The listing builds one solid part. Answer for the finished solid, in the listing's coordinates (mm). Face numbers are marked on the shaded views. A direction names the side the tool comes from. Round coordinates to 2 decimals unless told otherwise and drop trailing zeros. Loops run counter-clockwise (first coordinate to the right, second up) from the corner with the lowest first, then second, coordinate; pieces in that order, holes last. Notation, with made-up numbers: (19, -20.75) -> (52, -20.75) arc R30 ccw to (52, 4.25) -> close; hole circle Ø7 at (-1, 78). An arc over 180 degrees is marked (long way). One line per question, with ' | ' between items.
from build123d import *

# Parameters (mm, degrees)
SKETCH5_R           = 30
BOSS_EXTRUDE1_DEPTH = 5
SKETCH6_R           = 5.75
CUT_EXTRUDE1_DEPTH  = 50
SKETCH11_R          = 1.5
CUT_EXTRUDE2_DEPTH  = 43.720018727
SKETCH13_R          = 1.5
CUT_EXTRUDE3_DEPTH  = 10
CIRPATTERN2_COUNT   = 6
CUT_EXTRUDE4_DEPTH  = 10


with BuildPart() as part:
    # Sketch5 → Boss-Extrude1 (new body)
    with BuildSketch(Plane(origin=(0, 0, 0), x_dir=(1, 0, 0), z_dir=(0, 1, 0))):
        with Locations(Location((0, 0, 0), (0, 0, 270))):
            Circle(SKETCH5_R)
    extrude(amount=BOSS_EXTRUDE1_DEPTH)

    # Sketch6 → Cut-Extrude1 (cut)
    with BuildSketch(Plane(origin=(0, 5, 0), x_dir=(1, 0, 0), z_dir=(0, 1, 0))):
        with Locations(Location((5.564652455, 9.430649132, 0), (0, 0, 270))):
            Circle(SKETCH6_R)
        with Locations(Location((5.325305202, -9.567843252, 0), (0, 0, 270))):
            Circle(SKETCH6_R)
        with Locations(Location((-11.00819821, 0.138683741, 0), (0, 0, 270))):
            Circle(SKETCH6_R)
    extrude(amount=-CUT_EXTRUDE1_DEPTH, mode=Mode.SUBTRACT)

    # Sketch11 → Cut-Extrude2 (cut, through all)
    with BuildSketch(Plane(origin=(0, 5, 0), x_dir=(1, 0, 0), z_dir=(0, 1, 0))):
        with Locations(Location((0, 0, 0), (0, 0, 270))):
            Circle(SKETCH11_R)
    extrude(amount=-CUT_EXTRUDE2_DEPTH, mode=Mode.SUBTRACT)

    # Sketch13 → Cut-Extrude3 (cut)
    with BuildSketch(Plane(origin=(0, 5, 0), x_dir=(1, 0, 0), z_dir=(0, 1, 0))):
        with Locations(Location((0, 25, 0), (0, 0, 270))):
            Circle(SKETCH13_R)
    cut_extrude3 = extrude(amount=-CUT_EXTRUDE3_DEPTH, mode=Mode.SUBTRACT)

    # CirPattern2: Cut-Extrude3 ×6 about axis
    cirpattern2_axis = Axis((0, 0, 0), (0, 1, 0))
    for i in range(1, CIRPATTERN2_COUNT):
        add(cut_extrude3.rotate(cirpattern2_axis, i * 360 / CIRPATTERN2_COUNT), mode=Mode.SUBTRACT)

    # Sketch14 → Cut-Extrude4 (cut)
    with BuildSketch(Plane(origin=(0, 5, 0), x_dir=(1, 0, 0), z_dir=(0, 1, 0))):
        with BuildLine():
            Line((9.868938528, -7.038931193), (19.133510592, -23.684357125))
            ThreePointArc((19.133510592, -23.684357125), (17.118789327, -30.75690251), (10.046243942, -28.742181244))
            Line((10.046243942, -28.742181244), (0.781671877, -12.096755312))
            ThreePointArc((0.781671877, -12.096755312), (2.796393143, -5.024209927), (9.868938528, -7.038931193))
        make_face()
        with BuildLine():
            Line((1.086170675, 12.073223814), (10.767141384, 28.479969565))
            ThreePointArc((10.767141384, 28.479969565), (17.888197845, 30.315876663), (19.724104943, 23.194820202))
            Line((19.724104943, 23.194820202), (10.043134234, 6.788074451))
            ThreePointArc((10.043134234, 6.788074451), (2.922077773, 4.952167353), (1.086170675, 12.073223814))
        make_face()
        with BuildLine():
            Line((-10.970227288, -5.061177624), (-29.962029078, -5.199861364))
            ThreePointArc((-29.962029078, -5.199861364), (-35.199861364, -0.037970922), (-30.037970922, 5.199861364))
            Line((-30.037970922, 5.199861364), (-11.046169132, 5.338545105))
            ThreePointArc((-11.046169132, 5.338545105), (-5.808336846, 0.176654663), (-10.970227288, -5.061177624))
        make_face()
    extrude(amount=-CUT_EXTRUDE4_DEPTH, mode=Mode.SUBTRACT)


solid = part.part
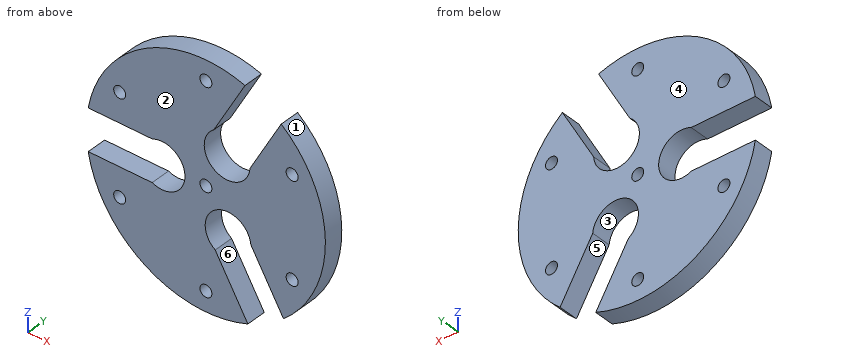
Q1. Find the intervals of material crossed by line 1 (Z direction, x = -21.5, y = 2.45); line 2 (X direction, y = 1.25, z = 12.5); line 3 (Z direction, x = 6, y = 3.45), in increasing order. Write a range as from..to.
Numbers:
line 1: -20.92..-13.99, -11.01..-5.26, 5.14..11.01, 13.99..20.92 | line 2: -27.27..-23.15, -20.15..0.38, 12.91..20.15, 23.15..27.27 | line 3: -29.39..-20.4, -3.7..3.86, 21.47..29.39
Q2. Given pin 1 Ø9 at (x, z) = (5.33, 9.57) entering from -Y; pin 2 Ø1.5 at (y, z) = (3.5, 17) entering from +X; pin 3 Ø1.5 at (y, z) = (4.5, -10) entering from +X; pin 4 Ø1.5 at (x, y) = (-4, 4) entering from -Z, each flat-ended and moving along its own axis, determine where each tip first touches the part or whether it passes through.
Numbers:
pin 1: through | pin 2: x = 25.22 | pin 3: x = 28.54 | pin 4: z = -29.82
Q3. A cutting plane is placed at D-D on y = 2.1. Give the vertices of the cut face in (x, z).
Numbers:
outline: (-29.55, -5.2) arc R30 ccw to (10.54, -28.09) -> (2.33, -14.19) arc R5.75 cw (long way) to (11.29, -8.9) -> (19.49, -22.8) arc R30 ccw to (18.91, 23.29) -> (11.06, 9.18) arc R5.75 cw (long way) to (1.98, 14.24) -> (9.83, 28.35) arc R30 ccw to (-29.55, 5.2) -> (-13.42, 5.08) arc R5.75 cw (long way) to (-13.5, -5.32) -> close; hole circle Ø3 at (-21.65, -12.5); hole circle Ø3 at (-21.65, 12.5); hole circle Ø3 at (0, -25); hole circle Ø3 at (0, 0); hole circle Ø3 at (0, 25); hole circle Ø3 at (21.65, -12.5); hole circle Ø3 at (21.65, 12.5)
Q4. A cutting plane is placed at C-C on z = 12.5. Give the vertices of the cut face in (x, y).
Numbers:
outline: (-27.27, 0) -> (-23.15, 0) -> (-23.15, 5) -> (-27.27, 5) -> close; (-20.15, 0) -> (0.38, 0) -> (0.38, 5) -> (-20.15, 5) -> close; (12.91, 0) -> (20.15, 0) -> (20.15, 5) -> (12.91, 5) -> close; (23.15, 0) -> (27.27, 0) -> (27.27, 5) -> (23.15, 5) -> close
Q5. A cutting plane is placed at B-B on x = -10. Give the vertices of the cut face in (y, z), plus the area to 3 significant figures.
Numbers:
outline: (0, -28.28) -> (5, -28.28) -> (5, -5.8) -> (0, -5.8) -> close; (0, 5.52) -> (5, 5.52) -> (5, 28.28) -> (0, 28.28) -> close | area: 226 mm^2
Q6. For the marked faces 4, 5 and 6, determine the directions among +Z, -Z, +X, -X, +Y, -Y from which every point of the face is accessible in a straight line to the end or side of a thin tool.
Numbers:
face 4: +Z, -Z, +X, -X, +Y | face 5: -Z, +Y, -Y | face 6: +Y, -Y
Q7. For a pull along Z with two mould halves and no side action, classify the marked faces 1, 2 and 3 as pulls with the +Z half, pulls with the -Z half, needs draft (parallel to the pull), parting line crosses it, or undercut.
Numbers:
face 1: parting line crosses it | face 2: needs draft | face 3: undercut
Q8. A cutting plane is placed at A-A on z = -10. Give the vertices of the cut face in (x, y), plus the area to 3 significant figures.
Numbers:
outline: (-28.28, 0) -> (-0.16, 0) -> (-0.16, 5) -> (-28.28, 5) -> close; (11.94, 0) -> (28.28, 0) -> (28.28, 5) -> (11.94, 5) -> close | area: 222 mm^2
